```python
from build123d import *

# Parameters (mm, degrees)
BOSS_EXTRUDE1_DEPTH = 488.95
SKETCH3_W           = 2.54
SKETCH3_H           = 2.032


with BuildPart() as part:
    # Sketch1 → Boss-Extrude1 (new body)
    with BuildSketch(Plane(origin=(0, 0, 0), x_dir=(1, 0, 0), z_dir=(0, 1, 0))):
        Polygon((7.332348419, 0), (3.666174209, 6.35), (-3.666174209, 6.35), (-7.332348419, 0), (-3.666174209, -6.35), (3.666174209, -6.35), align=None)
        Polygon((1.443375673, 2.5), (-1.443375673, 2.5), (-2.886751346, 0), (-1.443375673, -2.5), (1.443375673, -2.5), (2.886751346, 0), align=None, mode=Mode.SUBTRACT)
    extrude(amount=BOSS_EXTRUDE1_DEPTH)

    # Sketch3 → Cut-Revolve2 (revolve, cut)
    with BuildSketch(Plane(origin=(0, 0, 0), x_dir=(0, 0, -1), z_dir=(1, 0, 0))):
        with Locations((6.2865, 83.566)):
            Rectangle(SKETCH3_W, SKETCH3_H)
        with Locations((6.2865, 33.909)):
            Rectangle(SKETCH3_W, SKETCH3_H)
    revolve(axis=Axis((0, 488.95, 0), (0, -1, 0)), mode=Mode.SUBTRACT)


solid = part.part
```
Geometry check sheet. Reference: the model listing, model coordinates, mm. A direction names the side the tool comes from. Round coordinates to 2 decimals unless told otherwise and drop trailing zeros. Loops run counter-clockwise (first coordinate to the right, second up) from the corner with the lowest first, then second, coordinate; pieces in that order, holes last. Notation, with made-up numbers: (88.25, 78) -> (105.25, 78) arc R11 ccw to (105.25, 94) -> close; hole circle Ø2 at (4, 69.5). An arc over 180 degrees is marked (long way). Use a Markdown table: item, result.
(1) Sectioned sample at A-A (y = 175). Enter the section's corners in (x, z), then the cut area to 3 significant figures.
Calculated:
| item | result |
|---|---|
| outline | (-7.33, 0) -> (-3.67, -6.35) -> (3.67, -6.35) -> (7.33, 0) -> (3.67, 6.35) -> (-3.67, 6.35) -> close; hole (-2.89, 0) -> (-1.44, -2.5) -> (1.44, -2.5) -> (2.89, 0) -> (1.44, 2.5) -> (-1.44, 2.5) -> close |
| area | 118 mm² |
(2) Scan lines: probe 1 along Y at (x, z) = (-6, 1.75) (3 decimals); probe 2 along Z at (x, y) = (-2, 131.5); probe 3 along Z at (x, y) = (-0.75, 399). Record each from-to range of solid material in increasing order.
Calculated:
| item | result |
|---|---|
| probe 1 | 0 to 32.893, 34.925 to 82.55, 84.582 to 488.95 |
| probe 2 | -6.35 to -1.54, 1.54 to 6.35 |
| probe 3 | -6.35 to -2.5, 2.5 to 6.35 |
(3) Set-up check for faces 1 (the cylindrical face through (-3.052, 33.923, 3.981)), 2 (the flat face through (3.2, 0, -0.1)): record each of +Z, -Z, +X, -X, +Y, -Y from which the full face is reachable in a straight line by a thin tool's end or side.
Calculated:
| item | result |
|---|---|
| face 1 | none |
| face 2 | +Z, -Z, +X, -X, -Y |
(4) Go/stop test with flat-tipped pins: P1, Ø2, axis at x = 4, y = 199, coming from the -Z side; P2, Ø6, axis at y = 311, z = 1.5, coming from the +X side. Record where each tip stops, or that it passes through.
Calculated:
| item | result |
|---|---|
| P1 | z = -6.35 |
| P2 | x = 7.33 |
